Source: CAD feature listing. Evaluate the final solid. Frame: model axes, mm. Coordinates: 2 decimals unless noted, no trailing zeros. Loops run counter-clockwise (first coordinate to the right, second up) from the corner with the lowest first, then second, coordinate; pieces in that order, holes last.
from build123d import *

# Parameters (mm, degrees)
SKETCH_1_R        = 40
EXTRUDE_1_DEPTH   = 40
FILLET_1_R        = 2
SWEEP_3_PROFILE_R = 0.75
SKETCH_2_W        = 0.5
SKETCH_2_H        = 1


with BuildPart() as part:
    # 草图1 → 凸台-拉伸1 (new body)
    with BuildSketch(Plane(origin=(0, 0, 0), x_dir=(1, 0, 0), z_dir=(0, 1, 0))):
        Circle(SKETCH_1_R)
    extrude(amount=EXTRUDE_1_DEPTH)

    # 圆角1
    fillet_1_edges = [part.edges().sort_by_distance(p)[0] for p in [
        (-40, 40, 0),
    ]]
    fillet(fillet_1_edges, radius=FILLET_1_R)

    # 切除-扫描3: sweep along a path in 草图3
    with BuildLine(Plane.XZ) as sweep_3_path:
        CenterArc((0, 0), 9, 0, 360)
    # 切除-扫描3 profile (on start of the path) → 切除-扫描3 (sweep, cut)
    with BuildSketch(Plane(origin=(9, 0, 0), x_dir=(1, 0, 0), z_dir=(0, 0, 1))):
        Circle(SWEEP_3_PROFILE_R)
    sweep(path=sweep_3_path.line, mode=Mode.SUBTRACT)

    # 草图2 → 切除-旋转1 (revolve, cut)
    with BuildSketch(Plane.XY):
        with Locations((0.25, 0.5)):
            Rectangle(SKETCH_2_W, SKETCH_2_H)
    revolve(axis=Axis((0, 0, 0), (0, 1, 0)), mode=Mode.SUBTRACT)


solid = part.part
Q1. Line query: line 1 along Z through (x, y) = (0, 0.3); line 2 along Z through (x, y) = (0, 0.85); line 3 along Z through (x, y) = (0, 0.5). Output: solid intervals per line, ascending.
Q2. Contact query for flat-ended pins moving along their axis: pin 1 Ø3 at (x, y) = (-8.5, 32) entering from +Z; pin 2 Ø3 at (x, y) = (-9.5, 23) entering from -Z; pin 3 Ø4 at (x, y) = (11.5, 30) entering from -Z. Output: stop coordinate, or through.
Q3. Section A-A, the plane y = 29. Return the cut outline in (x, z).
Derived:
1. line 1: z = -40 to -9.69, -8.31 to -0.5, 0.5 to 8.31, 9.69 to 40
1. line 2: z = -40 to -0.5, 0.5 to 40
1. line 3: z = -40 to -9.56, -8.44 to -0.5, 0.5 to 8.44, 9.56 to 40
2. pin 1: stops at z = 39.38
2. pin 2: stops at z = -39.19
2. pin 3: stops at z = -38.86
3. outline: circle Ø80 at (0, 0)
